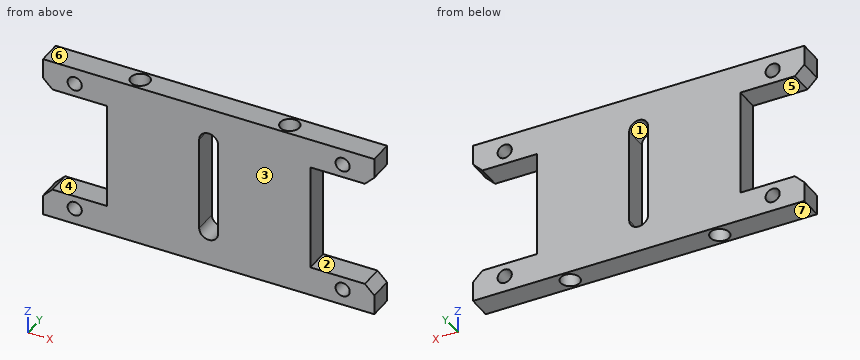
from build123d import *

# Parameters (mm, degrees)
SKETCH_1_R          = 1.5
EXTRUDE_1_DEPTH     = 5
CHAMFER_1_SIZE      = 2
SKETCH_2_R          = 2
CUT_EXTRUDE_1_DEPTH = 50.749371855


with BuildPart() as part:
    # 草图1 → 凸台-拉伸1 (new body)
    with BuildSketch(Plane(origin=(0, 0, 0), x_dir=(1, 0, 0), z_dir=(0, 1, 0))):
        Polygon((35, 17.5), (-35, 17.5), (-35, 11.288596674), (-21.49999999, 11.288596674), (-21.49999999, -11.288596674), (-35, -11.288596674), (-35, -17.5), (35, -17.5), (35, -11.288596674), (21.49999999, -11.288596674), (21.49999999, 11.288596674), (35, 11.288596674), align=None)
        with Locations(Location((-28.303727501, -14.088596674, 0), (0, 0, 270))):
            Circle(SKETCH_1_R, mode=Mode.SUBTRACT)
        with Locations(Location((28.303727501, -14.088596674, 0), (0, 0, 270))):
            Circle(SKETCH_1_R, mode=Mode.SUBTRACT)
        with BuildLine():
            ThreePointArc((-2, 10), (0, 12), (2, 10))
            Line((2, 10), (2, -10))
            ThreePointArc((2, -10), (0, -12), (-2, -10))
            Line((-2, -10), (-2, 10))
        make_face(mode=Mode.SUBTRACT)
        with Locations(Location((-28.303727501, 14.088596674, 0), (0, 0, 270))):
            Circle(SKETCH_1_R, mode=Mode.SUBTRACT)
        with Locations(Location((28.303727501, 14.088596674, 0), (0, 0, 270))):
            Circle(SKETCH_1_R, mode=Mode.SUBTRACT)
    extrude(amount=EXTRUDE_1_DEPTH)

    # 倒角1
    chamfer_1_edges = [part.edges().sort_by_distance(p)[0] for p in [
        (35, 2.5, 11.288596674),
        (-35, 2.5, 11.288596674),
        (-35, 2.5, -11.288596674),
        (35, 2.5, -11.288596674),
    ]]
    chamfer(chamfer_1_edges, length=CHAMFER_1_SIZE)

    # 草图2 → 切除-拉伸1 (cut, through all)
    with BuildSketch(Plane.XY.offset(17.5)):
        with Locations((-15.8, 2.5)):
            Circle(SKETCH_2_R)
        with Locations(Location((15.8, 2.5, 0), (0, 0, 180))):
            Circle(SKETCH_2_R)
    extrude(amount=-CUT_EXTRUDE_1_DEPTH, mode=Mode.SUBTRACT)


solid = part.part
Input: part model. Units: mm. Frame: model coordinates. Face numbers are marked on the shaded views. A direction names the side the tool comes from. Give positions to 0.01 mm unless a question says otherwise; leave off trailing zeros. Write each loop counter-clockwise with the first axis right and the second up, starting at its lowest first coordinate (ties: lowest second). Pieces come first, ordered by that corner, then holes. Notation, with made-up numbers: (60.25, -13) -> (85.25, -13) arc R35 cw to (85.25, 22) -> close; hole circle Ø7 at (-34, 83.5). An arc over 180 degrees is marked (long way). Use one line per item in the form item = value. Start each with the question number.
1) Section query C-C on y = 2.5. Count the separate pieces of the cut face and the enclosed holes in it, then the cut area to 3 significant figures.
2) Set-up query: the marked faces 1, 2, 3 and 4. Return all of +Z, -Z, +X, -X, +Y, -Y with unobstructed straight access to the full face (end or side cutting, diameter ignored); none if empty.
3) Pin query (flat end, axial travel): pin 1 (2.5 mm diameter, centred on y = 2.5, z = 3, fed in from +X). Return the tip coordinate at first contact, or that it passes through.
4) Draft query along Z for the marked faces 5, 6 and 7. Return one class per face: pulls with the +Z half, pulls with the -Z half, needs draft (parallel to the pull), parting line crosses it, or undercut.
5) Section query D-D on x = -24.5. Return the cut outline in (y, z).
6) Section query B-B on z = 6. Return the cut outline in (x, y).
7) Section query A-A on x = -17. Return the cut outline in (y, z), then the cut area to 3 significant figures.
8) Ray query, probe 1 along X at (y, z) = (2.35, -2); probe 2 along X at (y, z) = (3.05, 2); probe 3 along Z at (x, y) = (25.5, 1.6). Return the intervals inside material, ascending. Write a range as from..to.
Outcome:
q1.separate_pieces = 3
q1.enclosed_holes = 5
q1.area = 1,430 mm^2
q2.face_1 = +Y, -Y
q2.face_2 = +X, +Y, -Y
q2.face_3 = +Z, -Z, +X, -X, -Y
q2.face_4 = -X, +Y, -Y
q3.pin_1 = 21.5
q4.face_5 = undercut
q4.face_6 = pulls with the +Z half
q4.face_7 = pulls with the -Z half
q5.outline = (0, -17.5) -> (5, -17.5) -> (5, -11.29) -> (0, -11.29) -> close; (0, 11.29) -> (5, 11.29) -> (5, 17.5) -> (0, 17.5) -> close
q6.outline = (-21.5, 0) -> (-2, 0) -> (-2, 5) -> (-21.5, 5) -> close; (2, 0) -> (21.5, 0) -> (21.5, 5) -> (2, 5) -> close; hole circle Ø4 at (-15.8, 2.5); hole circle Ø4 at (15.8, 2.5)
q7.outline = (0, -17.5) -> (0.9, -17.5) -> (0.9, 17.5) -> (0, 17.5) -> close; (4.1, -17.5) -> (5, -17.5) -> (5, 17.5) -> (4.1, 17.5) -> close
q7.area = 63.0 mm^2
q8.probe_1 = -21.5..-17.79, -13.81..-2, 2..13.81, 17.79..21.5
q8.probe_2 = -21.5..-17.72, -13.88..-2, 2..13.88, 17.72..21.5
q8.probe_3 = -17.5..-11.29, 11.29..17.5
